from build123d import *

# Parameters (mm, degrees)
CENTER_RING_R         = 22.225
CENTER_RING_R_2       = 15.875
CENTER_DEPTH          = 9.525
OUTER_R               = 98.425
OUTER_R_2             = 89.535
OUTER_RING_DEPTH      = 9.525
BEAM_START            = -25.456769
BEEAM_W               = 3.175
BEEAM_H               = 19.05
BEAM_DEPTH            = 67.366769
CIRPATTERN1_COUNT     = 6
FILLET1_R             = 7.62
SKETCH27_R            = 20.955
CUT_EXTRUDE3_DEPTH    = 1.27
CUT_EXTRUDE5_START    = -8.946312
SKETCH31_R            = 3.175
CUT_EXTRUDE5_DEPTH    = 8.946312
CIRPATTERN5_COUNT     = 6
BODY_MOVE_COPY7_ANGLE = 31


with BuildPart() as part:
    # Center Ring → Center (new body, symmetric)
    with BuildSketch(Plane(origin=(0, 0, 0), x_dir=(1, 0, 0), z_dir=(0, 1, 0))):
        Circle(CENTER_RING_R)
        Circle(CENTER_RING_R_2, mode=Mode.SUBTRACT)
    extrude(amount=CENTER_DEPTH, both=True)



with BuildPart() as body_2:
    # Outer → Outer Ring (new body, symmetric)
    with BuildSketch(Plane(origin=(0, 0, 0), x_dir=(1, 0, 0), z_dir=(0, 1, 0))):
        Circle(OUTER_R)
        Circle(OUTER_R_2, mode=Mode.SUBTRACT)
    extrude(amount=OUTER_RING_DEPTH, both=True)


with BuildPart() as part_1:
    add(part.part)

    add(body_2.part)  # Beam merges body 2
    # beeam → Beam (add)
    with BuildSketch(Plane.XY.offset(47.625).offset(BEAM_START)):
        Rectangle(BEEAM_W, BEEAM_H)
    beam = extrude(amount=BEAM_DEPTH)

    # CirPattern1: Beam ×6 about axis
    cirpattern1_axis = Axis((0, 0, 0), (0, 1, 0))
    for i in range(1, CIRPATTERN1_COUNT):
        add(beam.rotate(cirpattern1_axis, i * 360 / CIRPATTERN1_COUNT))

    # Fillet1
    fillet1_edges = [part_1.edges().sort_by_distance(p)[0] for p in [
        (-1.5875, 0, 22.168231),
        (-1.5875, 0, 89.520925312),
        (1.5875, 0, 22.168231),
        (1.5875, 0, 89.520925312),
        (-18.404501203, 0, 12.458930829),
        (-76.733645491, 0, 46.135277985),
        (-19.992001203, 0, 9.709300171),
        (-78.321145491, 0, 43.385647328),
        (-19.992001203, 0, -9.709300171),
        (-78.321145491, 0, -43.385647328),
        (-18.404501203, 0, -12.458930829),
        (-76.733645491, 0, -46.135277985),
        (1.5875, 0, -22.168231),
        (1.5875, 0, -89.520925312),
        (-1.5875, 0, -22.168231),
        (-1.5875, 0, -89.520925312),
        (19.992001203, 0, -9.709300171),
        (78.321145491, 0, -43.385647328),
        (18.404501203, 0, -12.458930829),
        (76.733645491, 0, -46.135277985),
        (18.404501203, 0, 12.458930829),
        (76.733645491, 0, 46.135277985),
        (19.992001203, 0, 9.709300171),
        (78.321145491, 0, 43.385647328),
    ]]
    fillet(fillet1_edges, radius=FILLET1_R)

    # Sketch27 → Cut-Extrude3 (cut)
    with BuildSketch(Plane(origin=(0, 9.525, 0), x_dir=(1, 0, 0), z_dir=(0, 1, 0))):
        Circle(SKETCH27_R)
    extrude(amount=-CUT_EXTRUDE3_DEPTH, mode=Mode.SUBTRACT)

    # Sketch31 → Cut-Extrude5 (cut)
    with BuildSketch(Plane(origin=(49.2125, 0, 85.238550367), x_dir=(0, -1, 0), z_dir=(0.5, 0, 0.866025404)).offset(CUT_EXTRUDE5_START)):
        Circle(SKETCH31_R)
    cut_extrude5 = extrude(amount=CUT_EXTRUDE5_DEPTH, mode=Mode.SUBTRACT)

    # CirPattern5: Cut-Extrude5 ×6 about axis
    cirpattern5_axis = Axis((0, 9.525, 0), (0, -1, 0))
    for i in range(1, CIRPATTERN5_COUNT):
        add(cut_extrude5.rotate(cirpattern5_axis, i * 360 / CIRPATTERN5_COUNT), mode=Mode.SUBTRACT)


with BuildPart() as part_2:
    # Body-Move/Copy7: moved
    add(part_1.part.rotate(Axis((0, 0, 0), (0, -1, 0)), BODY_MOVE_COPY7_ANGLE))


solid = part_2.part
Work out the finished part from the listing and answer in its coordinate system (mm). A direction names the side the tool comes from. Give positions to 0.01 mm unless a question says otherwise; leave off trailing zeros. Loops run counter-clockwise (first coordinate to the right, second up) from the corner with the lowest first, then second, coordinate; pieces in that order, holes last. Notation, with made-up numbers: (70, -27.5) -> (100, -27.5) arc R25 ccw to (100, -12.5) -> close; hole circle Ø8 at (26.5, 23). An arc over 180 degrees is marked (long way). Use a Markdown table: item, result. Add a question column.
1. Find the intervals of material crossed by probe 1 along Z at (x, y) = (0, 4.25) (3 decimals); probe 2 along Z at (x, y) = (0, 8.6) (3 decimals); probe 3 along X at (y, z) = (4.5, -16), in increasing order.
2. Section B-B on x = 66.5 is taken. Determine the outline of the cut face in (y, z) (1 decimal), and give its area (3 significant figures).
3. For faces 4 (the cylindrical face through (-82.1, 0.413, -45.658)), 5 (the cylindrical face through (-2.08, -4.37, 89.51)), determine the directions among +Z, -Z, +X, -X, +Y, -Y from which every point of the face is accessible in a straight line to the end or side of a thin tool.
4. Determine the mould class of faces 1 (the cylindrical face through (80.97, -3.03, 47.54)), 2 (the flat face through (14, 8.255, -8)), 3 (the cylindrical face through (-48.48, -0.13, 72.53)) for opening direction Y: released by +Y, released by -Y, zero draft, split by the parting line, or undercut.
5. Flat-ended cylindrical pins translate along their axes: pin 1 Ø1.5 at (y, z) = (-4, 72) entering from -X; pin 2 Ø10 at (y, z) = (2.5, -47.5) entering from +X; pin 3 Ø10 at (x, y) = (-20, 3) entering from -Z; pin 4 Ø12.5 at (x, z) = (-5.5, 2.5) entering from +Y. Find the tip coordinate at first contact, or state that the pin passes through.
6. Section A-A on x = -68.5 is taken. Determine the outline of the cut face in (y, z) (3 decimals).
7. Section C-C on y = -7 is taken. State how many separate pieces and enclosed holes the cut face has, and give its area (3 significant figures).
Results below:
| question | item | result |
|---|---|---|
| 1 | probe 1 | z = -98.425 to -89.535, -22.225 to -15.875, 15.875 to 22.225, 89.535 to 98.425 |
| 1 | probe 2 | z = -98.425 to -89.535, -22.225 to -20.955, 20.955 to 22.225, 89.535 to 98.425 |
| 1 | probe 3 | x = -97.12 to -88.09, -15.57 to 15.79, 88.09 to 97.12 |
| 2 | outline | (-9.5, -72.6) -> (9.5, -72.6) -> (9.5, -60) -> (-9.5, -60) -> close; (-9.5, -0.4) -> (9.5, -0.4) -> (9.5, 2.7) -> (-9.5, 2.7) -> close; (-9.5, 60) -> (9.5, 60) -> (9.5, 72.6) -> (-9.5, 72.6) -> close |
| 2 | area | 541 mm^2 |
| 3 | face 4 | none |
| 3 | face 5 | +Y, -Y |
| 4 | face 1 | undercut |
| 4 | face 2 | released by +Y |
| 4 | face 3 | zero draft |
| 5 | pin 1 | stops at x = -67.9 |
| 5 | pin 2 | stops at x = 88.78 |
| 5 | pin 3 | stops at z = -97.28 |
| 5 | pin 4 | passes through |
| 6 | outline | (-9.525, -70.677) -> (9.525, -70.677) -> (9.525, -57.656) -> (-9.525, -57.656) -> close; (-9.525, -2.783) -> (9.525, -2.783) -> (9.525, 0.392) -> (-9.525, 0.392) -> close; (-9.525, 57.656) -> (9.525, 57.656) -> (9.525, 70.677) -> (-9.525, 70.677) -> close |
| 7 | separate pieces | 1 |
| 7 | enclosed holes | 7 |
| 7 | area | 7,550 mm^2 |
